```python
from build123d import *

# Parameters (mm, degrees)
F0_R     = 24.8703157221
F1_DEPTH = 32.512
F2_DEPTH = 11.684
F3_R     = 3.302


with BuildPart() as f1:
    # F0 (on Top) → F1 (new body)
    with BuildSketch(Plane.XY):
        with BuildLine():
            ThreePointArc((-14.4067881156, -28.1265414802), (2.4665893818, -18.3362616868), (9.1255648255, 0))
            ThreePointArc((9.1255648255, 0), (2.4665893818, 18.3362616868), (-14.4067881156, 28.1265414802))
            ThreePointArc((-14.4067881156, 28.1265414802), (-48.0244351745, 0), (-14.4067881156, -28.1265414802))
        make_face()
        with Locations((-19.4494351745, 0)):
            Circle(F0_R, mode=Mode.SUBTRACT)
        with Locations((-19.4494351745, 0)):
            Circle(F0_R)
        with BuildLine():
            Line((0, 3.4105645027), (0, 0))
            Line((0, 0), (0, -3.4105645027))
            Line((0, -3.4105645027), (-5.5749728057, -3.4105645027))
            ThreePointArc((-5.5749728057, -3.4105645027), (-19.4494351745, -14.2875), (-33.3238975433, -3.4105645027))
            ThreePointArc((-33.3238975433, -3.4105645027), (-33.7369351745, 0), (-33.3238975433, 3.4105645027))
            ThreePointArc((-33.3238975433, 3.4105645027), (-19.4494351745, 14.2875), (-5.5749728057, 3.4105645027))
            Line((-5.5749728057, 3.4105645027), (0, 3.4105645027))
        make_face(mode=Mode.SUBTRACT)
    extrude(amount=F1_DEPTH)

    # F0 (on Top) → F2 (join)
    with BuildSketch(Plane.XY):
        with BuildLine():
            ThreePointArc((-14.4067881156, 28.1265414802), (2.4665893818, 18.3362616868), (9.1255648255, 0))
            ThreePointArc((9.1255648255, 0), (2.4665893818, -18.3362616868), (-14.4067881156, -28.1265414802))
            Line((-14.4067881156, -28.1265414802), (37.8873295314, -18.7510276535))
            ThreePointArc((37.8873295314, -18.7510276535), (53.5755648255, 0), (37.8873295314, 18.7510276535))
            Line((37.8873295314, 18.7510276535), (-14.4067881156, 28.1265414802))
        make_face()
        with BuildLine():
            ThreePointArc((24.3655648255, 0), (34.5255648255, 10.16), (44.6855648255, 0))
            ThreePointArc((44.6855648255, 0), (34.5255648255, -10.16), (24.3655648255, 0))
        make_face(mode=Mode.SUBTRACT)
        with BuildLine():
            ThreePointArc((-14.4067881156, -28.1265414802), (2.4665893818, -18.3362616868), (9.1255648255, 0))
            ThreePointArc((9.1255648255, 0), (2.4665893818, 18.3362616868), (-14.4067881156, 28.1265414802))
            ThreePointArc((-14.4067881156, 28.1265414802), (-48.0244351745, 0), (-14.4067881156, -28.1265414802))
        make_face()
        with Locations((-19.4494351745, 0)):
            Circle(F0_R, mode=Mode.SUBTRACT)
    extrude(amount=F2_DEPTH)

    # F3
    f3_edges = [f1.edges().sort_by_distance(p)[0] for p in [
        (-48.024435, 0, 32.512),
    ]]
    fillet(f3_edges, radius=F3_R)


solid = f1.part
```
Here's how the part is built. I have some questions about the finished solid (model axes, mm). A direction names the side the tool comes from. Coordinates: 2 decimals unless noted, no trailing zeros. Order: outer loops, then holes, each group sorted by start corner. A loop starts at its lowest first (then second) coordinate and runs counter-clockwise, first axis right, second up. Notation, with made-up numbers: M 18.25,28.5 L 40.25,28.5 A17 cw 40.25,39.5 Z; hole C -6.75,-32 d8. An arc over 180 degrees is marked long. Answer as a JSON object with one key per item and string values. Group by question number.
(1) For pin 1 (5 mm diameter, centred on y = 9.5, z = 11, fed in from -X); pin 2 (6 mm diameter, centred on x = -3, z = 11, fed in from +Y); pin 3 (3 mm diameter, centred on x = -2, z = 7, fed in from +Y), each with a flat end and sliding along its axis, tell me the tip position at first contact or that it passes through.
(2) Suppose I cut it at B-B, the plane x = 30. Please give me the cut outline in (y, z), then the cut area to 3 significant figures.
(3) I need wall thicknesses on probe 1 along Z at (x, y) = (19, -2.5); probe 2 along Y at (x, z) = (-1, 7.5); probe 3 along Y at (x, z) = (-11, 27.5). Which ranges of each line are inside material? Lowest first, please.
(4) Which directions (+Z, -Z, +X, -X, +Y, -Y) give clear straight access to the entire face, cutting with the end or side of a thin tool? Please do faces 1 (the face through (2, 0, 0)), 2 (the face through (-3, -3.411, 16)).
(5) Suppose I cut it at C-C, the plane y = 0. State how many separate pieces and enclosed holes the cut face has, then the cut area to 3 significant figures.
(6) Suppose I cut it at D-D, the plane x = 16. Please give me the cut outline in (y, z), then the cut area to 3 significant figures.
(7) If we mould it in two halves opening along Y, with no side actions, what happens to faces 3 (the face through (19, 0, 11.684)), 4 (the face through (11.4, -23.5, 5.8)), 5 (the face through (-3, 3.411, 16))? For each: released by +Y, released by -Y, zero draft, split by the parting line, or undercut.
Values found:
{
 "1": {"pin 1": "stops at x = -47.15", "pin 2": "stops at y = 26.62", "pin 3": "stops at y = 26.17"},
 "2": {"outline": "M -20.17,0 L -9.1,0 L -9.1,11.68 L -20.17,11.68 Z; M 9.1,0 L 20.17,0 L 20.17,11.68 L 9.1,11.68 Z", "area": "259 mm^2"},
 "3": {"probe 1": "z = 0 to 11.68", "probe 2": "y = -25.72 to -3.41, 3.41 to 25.72", "probe 3": "y = -27.3 to -11.52, 11.52 to 27.3"},
 "4": {"face 1": "-Z, +X, -X, +Y, -Y", "face 2": "+Z, -Z"},
 "5": {"separate pieces": "3", "enclosed holes": "0", "area": "1,040 mm^2"},
 "6": {"outline": "M -22.68,0 L 22.68,0 L 22.68,11.68 L -22.68,11.68 Z", "area": "530 mm^2"},
 "7": {"face 3": "zero draft", "face 4": "released by -Y", "face 5": "undercut"}
}
